from build123d import *

# Parameters (mm, degrees)
BOSS_EXTRUDE1_DEPTH = 10
SKETCH2_W           = 1
SKETCH2_H           = 9
CUT_EXTRUDE1_DEPTH  = 0.5
SKETCH4_W           = 4.5
SKETCH4_H           = 1
CUT_EXTRUDE4_DEPTH  = 0.25
SKETCH5_W           = 4.5
SKETCH5_H           = 1
CUT_EXTRUDE5_DEPTH  = 0.25
SKETCH6_R           = 3
CUT_EXTRUDE6_DEPTH  = 34.739405243


with BuildPart() as part:
    # Sketch1 → Boss-Extrude1 (new body)
    with BuildSketch(Plane.XY):
        with BuildLine():
            Line((0, 0), (-9.88076328, -17.388804358))
            ThreePointArc((-9.88076328, -17.388804358), (-7.065247876, -27.614892222), (3.160839988, -24.799376818))
            Line((3.160839988, -24.799376818), (13.041603269, -7.41057246))
            add(Edge.make_bspline(
                [(13.041603269, -7.41057246), (14.806349741, -3.203268527), (10.991774611, -1.261774485), (9.965646647, 2)],
                knots=[0, 0, 0, 0, 1, 1, 1, 1], degree=3))
            Line((9.965646647, 2), (9.965646647, 17))
            Line((9.965646647, 17), (14.856831388, 17))
            Line((14.856831388, 17), (14.856831388, 26))
            Line((14.856831388, 26), (-0.034353353, 26))
            Line((-0.034353353, 26), (-0.034353353, 15))
            Line((-0.034353353, 15), (-0.034353353, 5))
            Line((-0.034353353, 5), (0, 0))
        make_face()
    extrude(amount=BOSS_EXTRUDE1_DEPTH)

    # Sketch2 → Cut-Extrude1 (cut)
    with BuildSketch(Plane(origin=(14.856831388, 0, 0), x_dir=(0, 0, -1), z_dir=(1, 0, 0))):
        with Locations((-5, 21.5)):
            Rectangle(SKETCH2_W, SKETCH2_H)
    extrude(amount=-CUT_EXTRUDE1_DEPTH, mode=Mode.SUBTRACT)

    # Sketch4 → Cut-Extrude4 (cut)
    with BuildSketch(Plane(origin=(14.856831388, 0, 0), x_dir=(0, 0, -1), z_dir=(1, 0, 0))):
        with Locations((-7.75, 17.5)):
            Rectangle(SKETCH4_W, SKETCH4_H)
        with Locations((-7.75, 19.5)):
            Rectangle(SKETCH4_W, SKETCH4_H)
        with Locations((-7.75, 21.5)):
            Rectangle(SKETCH4_W, SKETCH4_H)
        with Locations((-7.75, 23.5)):
            Rectangle(SKETCH4_W, SKETCH4_H)
        with Locations((-7.75, 25.5)):
            Rectangle(SKETCH4_W, SKETCH4_H)
    extrude(amount=-CUT_EXTRUDE4_DEPTH, mode=Mode.SUBTRACT)

    # Sketch5 → Cut-Extrude5 (cut)
    with BuildSketch(Plane(origin=(14.856831388, 0, 0), x_dir=(0, 0, -1), z_dir=(1, 0, 0))):
        with Locations((-2.25, 17.5)):
            Rectangle(SKETCH5_W, SKETCH5_H)
        with Locations((-2.25, 19.5)):
            Rectangle(SKETCH5_W, SKETCH5_H)
        with Locations((-2.25, 21.5)):
            Rectangle(SKETCH5_W, SKETCH5_H)
        with Locations((-2.25, 23.5)):
            Rectangle(SKETCH5_W, SKETCH5_H)
        with Locations((-2.25, 25.5)):
            Rectangle(SKETCH5_W, SKETCH5_H)
    extrude(amount=-CUT_EXTRUDE5_DEPTH, mode=Mode.SUBTRACT)

    # Sketch6 → Cut-Extrude6 (cut, through all)
    with BuildSketch(Plane.XY.offset(10)):
        with Locations((-4.31940135, -22.782574446)):
            Circle(SKETCH6_R)
        with Locations((6.520801634, -3.70528623)):
            Circle(SKETCH6_R)
    extrude(amount=-CUT_EXTRUDE6_DEPTH, mode=Mode.SUBTRACT)


solid = part.part
Geometry check sheet. Reference: the model listing, model coordinates, mm. A direction names the side the tool comes from. Round coordinates to 2 decimals unless told otherwise and drop trailing zeros. Order: outer loops, then holes, each group sorted by start corner. A loop starts at its lowest first (then second) coordinate and runs counter-clockwise, first axis right, second up. Notation, with made-up numbers: M 75,72.5 L 102,72.5 A19 ccw 102,100.5 Z; hole C 32,31 d6. An arc over 180 degrees is marked long. Answer in a Markdown table with one row per item. Add a question column.
Item 1: Material ranges on L1, parallel to X at y = 10, z = 9; L2, parallel to Y at x = 5.25, z = 3.25; L3, parallel to Y at x = 5, z = 4, recorded low to high. Write a range as [from, to].
Item 2: Sectioned sample at B-B, the plane z = 7.5. State how many separate pieces and enclosed holes the cut face has, plus the area to 3 significant figures.
Item 3: Sectioned sample at D-D, the plane x = 5. Enter the section's corners in (y, z), plus the area to 3 significant figures.
Item 4: Set-up check for faces 4 (the face through (14.357, 22, 5)), 5 (the face through (14.607, 17.5, 2.3)), 6 (the face through (14.607, 25.5, 2.3)): record each of +Z, -Z, +X, -X, +Y, -Y from which the full face is reachable in a straight line by a thin tool's end or side.
Item 5: Depth check by flat-ended pin: pin 1 Ø0.8 at (y, z) = (25.5, 6.5) entering from +X; pin 2 Ø1 at (y, z) = (-6, 7) entering from +X; pin 3 Ø1.5 at (y, z) = (19.5, 2.5) entering from -X. Enter the tip coordinate at first touch or a pass-through.
Item 6: Sectioned sample at C-C, the plane y = 16. Enter the section's corners in (x, z), plus the area to 3 significant figures.
Item 7: Draft check along X on faces 1 (the face through (4.31, -1.68, 5.07)), 2 (the face through (14.857, 18.5, 2.2)), 3 (the face through (7, 26, 5)). Enter one of: released by +X, released by -X, zero draft, split by the parting line, or undercut.
Item 8: Sectioned sample at A-A, the plane x = -4.25. Enter the section's corners in (y, z).
Filled in:
| question | item | result |
|---|---|---|
| 1 | L1 | x = [-0.03, 9.97] |
| 1 | L2 | y = [-21.12, -6.42], [-0.99, 26] |
| 1 | L3 | y = [-21.56, -6.29], [-1.12, 26] |
| 2 | separate pieces | 1 |
| 2 | enclosed holes | 2 |
| 2 | area | 682 mm² |
| 3 | outline | M -21.56,0 L -6.29,0 L -6.29,10 L -21.56,10 Z; M -1.12,0 L 26,0 L 26,10 L -1.12,10 Z |
| 3 | area | 424 mm² |
| 4 | face 4 | +X, +Y, -Y |
| 4 | face 5 | +Z, -Z, +X, -Y |
| 4 | face 6 | +Z, -Z, +X, +Y |
| 5 | pin 1 | stops at x = 14.61 |
| 5 | pin 2 | stops at x = 13.5 |
| 5 | pin 3 | stops at x = -0.03 |
| 6 | outline | M -0.03,0 L 9.97,0 L 9.97,10 L -0.03,10 Z |
| 6 | area | 100 mm² |
| 7 | face 1 | undercut |
| 7 | face 2 | released by +X |
| 7 | face 3 | zero draft |
| 8 | outline | M -28.54,0 L -25.78,0 L -25.78,10 L -28.54,10 Z; M -19.78,0 L -7.48,0 L -7.48,10 L -19.78,10 Z |
